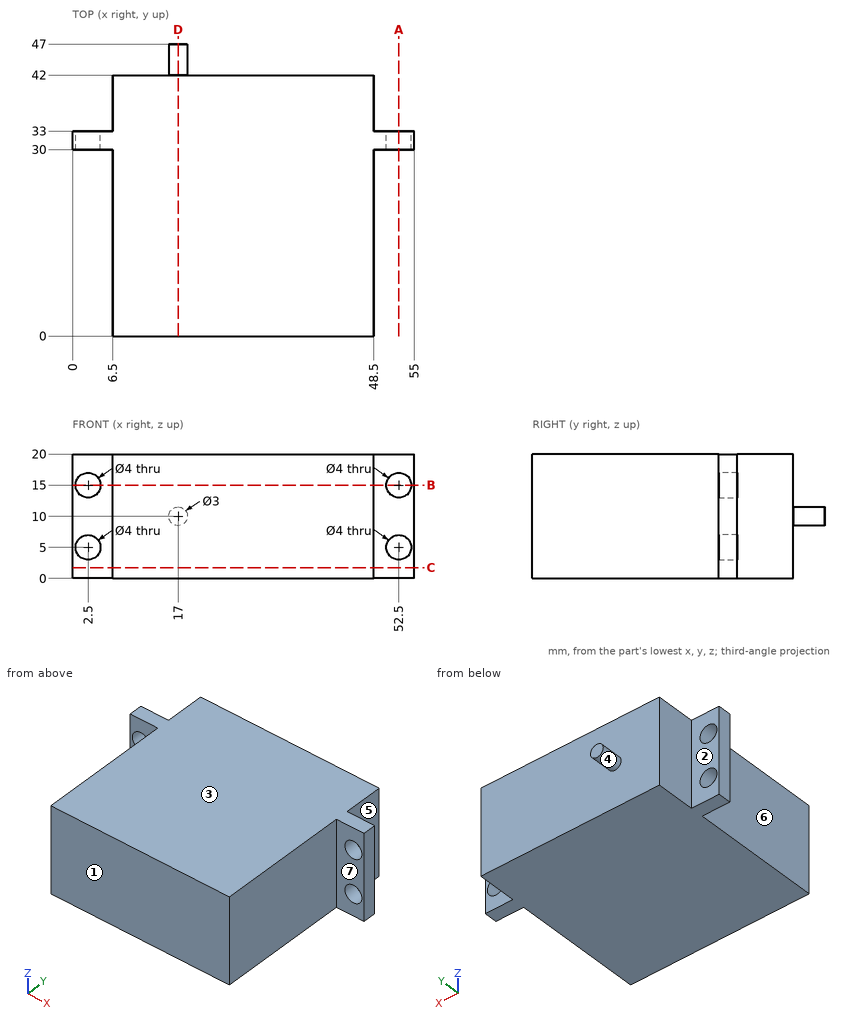
Answer from the drawing. Dimensions are ordinates in mm from the lowest x, y and z of the part. A direction names the side the tool comes from. Coordinates: 2 decimals unless noted, no trailing zeros. Write each loop counter-clockwise with the first axis right and the second up, starting at its lowest first coordinate (ties: lowest second). Pieces come first, ordered by that corner, then holes. Notation, with made-up numbers: (8, -5.5) - (48, -5.5) arc R23 cw to (48, 18.5) - close; hole circle Ø2 at (-12, 53.5). An arc over 180 degrees is marked (long way). Return JSON: item names as keys, results as strings. Group by question number.
Q1. For a pull along Y with two mould halves and no side action, classify the marked faces 1, 2 and 3 as +Y half, -Y half, draft (parallel to the pull), parting line (faces both ways), or undercut.
Q2. Flat-ended cylindrical pins translate along their axes: pin 1 Ø2.5 at (x, z) = (52.5, 15) entering from +Y; pin 2 Ø3 at (x, z) = (50.5, 7.5) entering from -Y; pin 3 Ø3 at (x, z) = (1.5, 7) entering from +Y; pin 4 Ø4 at (y, z) = (19.5, 16.5) entering from -X. Find the tip coordinate at first contact, or state that the pin passes through.
Q3. Find the intervals of material crossed by line 1 along X through (y, z) = (32, 5); line 2 along Z through (x, y) = (52, 31); line 3 along X through (y, z) = (32, 16.75), in increasing order. Write a range as [from, to].
Q4. The part is cut by section A-A on x = 52.5. Write down the section's boundary in (y, z).
Q5. The part is cut by section D-D on x = 17. Write down the section's boundary in (y, z).
Q6. The part is cut by section B-B on z = 15. Write down the section's boundary in (x, y).
Q7. Which of the six approach directions +Z, -Z, +X, -X, +Y, -Y give full straight-line access (tool end or side, diameter ignored) to the marked faces 4, 5, 6 and 7?
Q8. The part is cut by section C-C on z = 1.75. Write down the section's boundary in (x, y), and give its area (3 significant figures).
Evaluation:
{
 "1": {"face 1": "-Y half", "face 2": "+Y half", "face 3": "draft"},
 "2": {"pin 1": "passes through", "pin 2": "stops at y = 30", "pin 3": "stops at y = 33", "pin 4": "stops at x = 6.5"},
 "3": {"line 1": "x = [0, 0.5], [4.5, 50.5], [54.5, 55]", "line 2": "z = [0, 3.06], [6.94, 13.06], [16.94, 20]", "line 3": "x = [0, 1.53], [3.47, 51.53], [53.47, 55]"},
 "4": {"outline": "(30, 0) - (33, 0) - (33, 3) - (30, 3) - close; (30, 7) - (33, 7) - (33, 13) - (30, 13) - close; (30, 17) - (33, 17) - (33, 20) - (30, 20) - close"},
 "5": {"outline": "(0, 0) - (42, 0) - (42, 8.5) - (47, 8.5) - (47, 11.5) - (42, 11.5) - (42, 20) - (0, 20) - close"},
 "6": {"outline": "(0, 30) - (0.5, 30) - (0.5, 33) - (0, 33) - close; (4.5, 30) - (6.5, 30) - (6.5, 0) - (48.5, 0) - (48.5, 30) - (50.5, 30) - (50.5, 33) - (48.5, 33) - (48.5, 42) - (6.5, 42) - (6.5, 33) - (4.5, 33) - close; (54.5, 30) - (55, 30) - (55, 33) - (54.5, 33) - close"},
 "7": {"face 4": "+Y", "face 5": "+Z, -Z, +X, +Y", "face 6": "+Z, -Z, -X, -Y", "face 7": "+Z, -Z, +X, -Y"},
 "8": {"outline": "(0, 30) - (6.5, 30) - (6.5, 0) - (48.5, 0) - (48.5, 30) - (55, 30) - (55, 33) - (48.5, 33) - (48.5, 42) - (6.5, 42) - (6.5, 33) - (0, 33) - close", "area": "1,800 mm2"}
}
